Could you check a few things on this model? Use its own coordinates, in mm. Give positions to 0.01 mm unless a question says otherwise; leave off trailing zeros. Loops run counter-clockwise (first coordinate to the right, second up) from the corner with the lowest first, then second, coordinate; pieces in that order, holes last. Notation, with made-up numbers: (20, 30) - (58, 30) arc R20 ccw to (58, 58) - close; hole circle Ø11 at (44, -1.75). An arc over 180 degrees is marked (long way). Write each question's results on one line, items separated by ' | '. Start each with the question number.
(1) I need wall thicknesses on line 1 (Y direction, x = 40, z = 5); line 2 (Y direction, x = 14, z = -1); line 3 (Z direction, x = 61, y = 0). Which ranges of each line are inside material? Lowest first, please.
(2) If we mould it in two halves opening along Z, with no side actions, what happens to faces 1 (the face through (37.57, -25.5, 30.99)), 2 (the face through (37.567, -87.985, 39.163)), 3 (the face through (76.2, -54, 23))? For each: released by +Z, released by -Z, zero draft, split by the parting line, or undercut.
(3) Suppose I cut it at B-B (y = -82.5). Please give me the cut outline in (x, z), and give its area (3 significant figures).
(4) Suppose I cut it at C-C (z = 28). Please give me the cut outline in (x, y), and give its area (3 significant figures).
(5) For pin 1 (10 mm diameter, centred on x = 55, y = -55, fed in from -Z); pin 2 (1.5 mm diameter, centred on x = 14.5, z = 7, fed in from -Y); pin 3 (1 mm diameter, centred on x = 17.5, z = 49, fed in from -Y), each with a flat end and sliding along its axis, tell me the tip position at first contact or that it passes through.
(6) Suppose I cut it at A-A (x = 65). Please give me the cut outline in (y, z).
from build123d import *

# Parameters (mm, degrees)
F1_DEPTH = 76.2


with BuildPart() as f1:
    # F0 (on Right) → F1 (new body)
    with BuildSketch(Plane.YZ):
        with BuildLine():
            ThreePointArc((-50.8877843666, -26.1272218461), (-35.5301604305, -11.2844595025), (-15.2511948734, -17.9872770357))
            ThreePointArc((-15.2511948734, -17.9872770357), (-0.1647004468, -0.7373577806), (5.2721587586, 21.5247757733))
            ThreePointArc((5.2721587586, 21.5247757733), (5.2720026358, 21.6475777712), (5.2715342684, 21.7703789752))
            ThreePointArc((5.2715342684, 21.7703789752), (-25.7544503942, 31.4232390217), (-18.4018610728, 63.0733395213))
            ThreePointArc((-18.4018610728, 63.0733395213), (-88.4049130397, 38.0519285625), (-50.8877843666, -26.1272218461))
        make_face()
    extrude(amount=F1_DEPTH)


solid = f1.part
Output values:
1) line 1: -88.41 to 2.36 | line 2: -85.75 to -0.3 | line 3: -0.42 to 19.96
2) face 1: undercut | face 2: split by the parting line | face 3: zero draft
3) outline: (0, -6.3) - (76.2, -6.3) - (76.2, 49.35) - (0, 49.35) - close | area: 4,240 mm2
4) outline: (0, -90.88) - (76.2, -90.88) - (76.2, -23.37) - (0, -23.37) - close | area: 5,140 mm2
5) pin 1: z = -26.13 | pin 2: y = -89.31 | pin 3: y = -83.09
6) outline: (-50.89, -26.13) arc R20.64 cw to (-15.25, -17.99) arc R48.3 ccw to (5.27, 21.77) arc R23.87 cw to (-18.4, 63.07) arc R48.3 ccw (long way) to start
